Design review of the part built by this model. Coordinates are the model's own, in mm. A direction names the side the tool comes from. Give positions to 0.01 mm unless a question says otherwise; leave off trailing zeros. Order: outer loops, then holes, each group sorted by start corner. A loop starts at its lowest first (then second) coordinate and runs counter-clockwise, first axis right, second up. Notation, with made-up numbers: (0, 62.5) -> (18, 62.5) arc R29 ccw to (18, 100.5) -> close; hole circle Ø10 at (46.5, -16.75). An arc over 180 degrees is marked (long way). Return JSON: item names as keys, results as strings.
```python
from build123d import *

# Parameters (mm, degrees)
F1_DEPTH = 25.4
F2_DEPTH = 7.9375
F3_DEPTH = 63.5
F0_W     = 25.4
F0_H     = 19.05
F4_DEPTH = 25.4
F6_R     = 6.35


with BuildPart() as f1:
    # F0 (on Front) → F1 (new body, symmetric)
    with BuildSketch(Plane.XZ):
        with BuildLine():
            Line((22.225, 9.525), (41.275, 9.525))
            Line((41.275, 9.525), (41.275, 27.0847757391))
            ThreePointArc((41.275, 27.0847757391), (46.5190025255, 38.8744965881), (58.7864982926, 42.8752))
            Line((58.7864982926, 42.8752), (60.325, 42.8752))
            Line((60.325, 42.8752), (60.325, 61.9252))
            Line((60.325, 61.9252), (59.579086726, 61.9252))
            add(Edge.make_bspline(
                [(49.820043734, 61.2319186085), (53.2136012382, 61.6294074654), (56.4831276325, 61.8655861507), (59.5790867259, 61.9252)],
                knots=[104.2253932415, 104.2253932415, 104.2253932415, 104.2253932415, 113.6544225684, 113.6544225684, 113.6544225684, 113.6544225684], degree=3))
            ThreePointArc((49.820043734, 61.2319186085), (29.9861053272, 49.0365057667), (22.225, 27.0847757391))
            Line((22.225, 27.0847757391), (22.225, 9.525))
        make_face()
    extrude(amount=F1_DEPTH, both=True)

    # F0 (on Front) → F2 (join, symmetric)
    with BuildSketch(Plane.XZ):
        with BuildLine():
            Line((-41.275, 9.525), (22.225, 9.525))
            Line((22.225, 9.525), (22.225, 27.0847757391))
            ThreePointArc((22.225, 27.0847757391), (29.9861053272, 49.0365057667), (49.820043734, 61.2319186085))
            add(Edge.make_bspline(
                [(-41.275, 9.525), (-40.3570706701, 32.7350297492), (12.3087736869, 56.838207338), (49.820043734, 61.2319186085)],
                knots=[0, 0, 0, 0, 104.2253932415, 104.2253932415, 104.2253932415, 104.2253932415], degree=3))
        make_face()
    extrude(amount=F2_DEPTH, both=True)

    # F0 (on Front) → F3 (join, symmetric)
    with BuildSketch(Plane.XZ):
        Polygon((41.275, -9.525), (41.275, 9.525), (22.225, 9.525), (-41.275, 9.525), (-41.275, -9.525), align=None)
    extrude(amount=F3_DEPTH, both=True)

    # F0 (on Front) → F4 (join, symmetric)
    with BuildSketch(Plane.XZ):
        with Locations((73.025, 52.4002)):
            Rectangle(F0_W, F0_H)
    extrude(amount=F4_DEPTH, both=True)

    # F0 (on Front) → F5 (revolve)
    with BuildSketch(Plane.XZ):
        Polygon((85.725, 61.9252), (85.725, 42.8752), (85.725, 38.1), (111.125, 38.1), (111.125, 66.675), (85.725, 66.675), align=None)
    revolve(axis=Axis((85.725, 0, 54.7751), (0, 0, 1)))

    # F6
    f6_edges = [f1.edges().sort_by_distance(p)[0] for p in [
        (-41.275, -63.5, 0),
        (41.275, -63.5, 0),
        (-41.275, 63.5, 0),
        (41.275, 63.5, 0),
    ]]
    fillet(f6_edges, radius=F6_R)


solid = f1.part
```
Item 1: For pin 1 (11 mm diameter, centred on y = -8.5, z = 3, fed in from +X) (3 decimals); pin 2 (12 mm diameter, centred on x = 8.5, z = 48.5, fed in from +Y); pin 3 (16.5 mm diameter, centred on x = 4.5, y = 33.5, fed in from +Z) (3 decimals), all flat-tipped, find the tip position at first contact; note any pin that passes through.
Result set:
{"pin 1": "stops at x = 41.275", "pin 2": "stops at y = 7.94", "pin 3": "stops at z = 9.525"}
Item 2: Mouldability with a two-part tool opening along X and no side actions: class faces 1 (the face through (60, 0, 42.875)), 2 (the face through (-39.365, -61.689, -0.133)), 3 (the face through (1, 35, 9.525)) as released by +X, released by -X, zero draft, split by the parting line, or undercut.
Result set:
{"face 1": "undercut", "face 2": "released by -X", "face 3": "zero draft"}
Item 3: Wall thickness on L1, parallel to X at y = 25, z = -3.5 (3 decimals); L2, parallel to Y at x = 38.5, z = 36.5; L3, parallel to Z at x = 100, y = 18.5 (3 decimals): over which ranges is each line inside the solid? List them lowest first. Write a range as [from, to].
Result set:
{"L1": "x = [-41.275, 41.275]", "L2": "y = [-25.4, 25.4]", "L3": "z = [38.1, 66.675]"}
Item 4: Add section A-A (z = 5). Give the boundary of the cut face in (x, y) (3 decimals), plus the area to 3 significant figures.
Result set:
{"outline": "(-41.275, -57.15) arc R6.35 ccw to (-34.925, -63.5) -> (34.925, -63.5) arc R6.35 ccw to (41.275, -57.15) -> (41.275, 57.15) arc R6.35 ccw to (34.925, 63.5) -> (-34.925, 63.5) arc R6.35 ccw to (-41.275, 57.15) -> close", "area": "10,400 mm^2"}
Item 5: Machinability: for faces 4 (the face through (46, -25.4, 42)), 5 (the face through (22.225, -17, 18)), 6 (the face through (60, 0, 61.925)), which of the approach directions +Z, -Z, +X, -X, +Y, -Y give a long, thin tool a straight path to every point of the face, cutting with its end or side? Answer none if there is none.
Result set:
{"face 4": "+Z, +X, -X, -Y", "face 5": "+Z, -X, -Y", "face 6": "+Z, -X"}
Item 6: Add section B-B (y = -40). Give the boundary of the cut face in (x, z) (3 decimals).
Result set:
{"outline": "(-41.275, -9.525) -> (41.275, -9.525) -> (41.275, 9.525) -> (-41.275, 9.525) -> close"}
